For this review, take the finished solid that the model builds, in its own axes (mm). A direction names the side the tool comes from. Round coordinates to 2 decimals unless told otherwise and drop trailing zeros. Order: outer loops, then holes, each group sorted by start corner. A loop starts at its lowest first (then second) coordinate and runs counter-clockwise, first axis right, second up. Notation, with made-up numbers: M 88.5,-7 L 135.5,-7 A30 ccw 135.5,29 Z; hole C 0.25,31.5 d7. An arc over 180 degrees is marked long. Use a Markdown table: item, result.
from build123d import *

# Parameters (mm, degrees)
SKETCH1_R           = 37
BOSS_EXTRUDE1_DEPTH = 7
SKETCH2_R           = 36
CUT_EXTRUDE1_DEPTH  = 6
SKETCH3_R           = 18.5
CUT_EXTRUDE2_DEPTH  = 6
FILLET1_R           = 1


with BuildPart() as part:
    # Sketch1 → Boss-Extrude1 (new body)
    with BuildSketch(Plane(origin=(0, 0, 0), x_dir=(1, 0, 0), z_dir=(0, 1, 0))):
        Circle(SKETCH1_R)
    extrude(amount=BOSS_EXTRUDE1_DEPTH)

    # Sketch2 → Cut-Extrude1 (cut)
    with BuildSketch(Plane(origin=(0, 7, 0), x_dir=(1, 0, 0), z_dir=(0, 1, 0))):
        Circle(SKETCH2_R)
    extrude(amount=-CUT_EXTRUDE1_DEPTH, mode=Mode.SUBTRACT)

    # Sketch3 → Cut-Extrude2 (cut)
    with BuildSketch(Plane(origin=(0, 1, 0), x_dir=(1, 0, 0), z_dir=(0, 1, 0))):
        Circle(SKETCH3_R)
    extrude(amount=-CUT_EXTRUDE2_DEPTH, mode=Mode.SUBTRACT)

    # Fillet1
    fillet1_edges = [part.edges().sort_by_distance(p)[0] for p in [
        (-37, 0, 0),
        (-36, 1, 0),
    ]]
    fillet(fillet1_edges, radius=FILLET1_R)


solid = part.part
Q1. Draft analysis for pull direction Z (two halves, no side actions). For faces 3 (the flat face through (-17, 0, -9)), 4 (the cylindrical face through (-8.02, 3.96, 36.12)), 5 (the cylindrical face through (-4.01, 0.51, 18.06)), state which applies: pulls with the +Z half, pulls with the -Z half, needs draft (parallel to the pull), parting line crosses it, or undercut.
Determined:
| item | result |
|---|---|
| face 3 | needs draft |
| face 4 | parting line crosses it |
| face 5 | undercut |
Q2. Wall thickness on line 1 along X through (y, z) = (5, 0); line 2 along Y through (x, z) = (-7, 23): over which ranges is each line inside the solid? List them lowest first. Write a range as [from, to].
Determined:
| item | result |
|---|---|
| line 1 | x = [-37, -36], [36, 37] |
| line 2 | y = [0, 1] |
Q3. Machinability: for faces 1 (the flat face through (15, 1, 15)), 2 (the flat face through (8, 7, 35.5)), which of the approach directions +Z, -Z, +X, -X, +Y, -Y give a long, thin tool a straight path to every point of the face, cutting with its end or side? Answer none if there is none.
Determined:
| item | result |
|---|---|
| face 1 | +Y |
| face 2 | +Z, -Z, +X, -X, +Y |
Q4. Clearance check with flat-ended pins moving along their axes: pin 1 (8 mm diameter, centred on x = -10, z = 24.5, fed in from +Y); pin 2 (2 mm diameter, centred on y = 6, z = 3.5, fed in from +X); pin 3 (1 mm diameter, centred on x = 25.5, z = -1, fed in from -Y); pin 4 (2 mm diameter, centred on y = 5, z = -23, fed in from -X). State where each tip first meets the part, or that it passes through.
Determined:
| item | result |
|---|---|
| pin 1 | stops at y = 1 |
| pin 2 | stops at x = 36.92 |
| pin 3 | stops at y = 0 |
| pin 4 | stops at x = -29.75 |
Q5. Add section B-B (z = 0). Write out the cut boundary in (x, y), then the cut area to 3 significant figures.
Determined:
| item | result |
|---|---|
| outline | M -37,1 A1 ccw -36,0 L -18.5,0 L -18.5,1 L -35,1 A1 cw -36,2 L -36,7 L -37,7 Z; M 18.5,0 L 36,0 A1 ccw 37,1 L 37,7 L 36,7 L 36,2 A1 cw 35,1 L 18.5,1 Z |
| area | 49.0 mm^2 |
Q6. Add section A-A (x = 0). Write out the cut boundary in (y, z).
Determined:
| item | result |
|---|---|
| outline | M 0,-36 A1 ccw 1,-37 L 7,-37 L 7,-36 L 2,-36 A1 cw 1,-35 L 1,-18.5 L 0,-18.5 Z; M 0,18.5 L 1,18.5 L 1,35 A1 cw 2,36 L 7,36 L 7,37 L 1,37 A1 ccw 0,36 Z |
Q7. Add section C-C (y = 3.75). Write out the cut boundary in (x, z), then the cut area to 3 significant figures.
Determined:
| item | result |
|---|---|
| outline | C 0,0 d74; hole C 0,0 d72 |
| area | 229 mm^2 |
